Here's how the part is built. I have some questions about the finished solid (model axes, mm). Face numbers are marked on the shaded views. Round coordinates to 2 decimals unless told otherwise and drop trailing zeros. Loops run counter-clockwise (first coordinate to the right, second up) from the corner with the lowest first, then second, coordinate; pieces in that order, holes last. Notation, with made-up numbers: M 39,52 L 77,52 A32 cw 77,83 Z; hole C 43,-18.75 d1. An arc over 180 degrees is marked long. Use a Markdown table: item, result.
```python
from build123d import *

# Parameters (mm, degrees)
F1_W     = 78
F1_H     = 78
F1_R     = 2.3
F1_R_2   = 1.25
F2_DEPTH = 1.6
F3_W     = 17
F3_H     = 17
F3_R     = 2.3
F3_R_2   = 1.25
F4_DEPTH = 5.1
F5_DEPTH = 10
F6_SIZE  = 3
F7_R     = 3
F8_SIZE  = 4
F9_DEPTH = 12.5


with BuildPart() as f2:
    # F1 (on Top) → F2 (new body, symmetric)
    with BuildSketch(Plane.XY):
        Rectangle(F1_W, F1_H)
        with Locations((-36, -34.35)):
            Circle(F1_R, mode=Mode.SUBTRACT)
        with Locations((7.7, -34.35)):
            Circle(F1_R, mode=Mode.SUBTRACT)
        with Locations((36, -34.35)):
            Circle(F1_R, mode=Mode.SUBTRACT)
        with Locations((-36, 9.35)):
            Circle(F1_R, mode=Mode.SUBTRACT)
        with Locations((7.7, 9.35)):
            Circle(F1_R, mode=Mode.SUBTRACT)
        with Locations((36, 9.35)):
            Circle(F1_R, mode=Mode.SUBTRACT)
        with Locations((0, 25.5)):
            Circle(F1_R_2, mode=Mode.SUBTRACT)
        with Locations((-36, 9.35)):
            Circle(F1_R)
        with Locations((-36, 9.35)):
            Circle(F1_R_2, mode=Mode.SUBTRACT)
        with Locations((36, 9.35)):
            Circle(F1_R)
        with Locations((36, 9.35)):
            Circle(F1_R_2, mode=Mode.SUBTRACT)
        with Locations((36, -34.35)):
            Circle(F1_R)
        with Locations((36, -34.35)):
            Circle(F1_R_2, mode=Mode.SUBTRACT)
        with Locations((-36, -34.35)):
            Circle(F1_R)
        with Locations((-36, -34.35)):
            Circle(F1_R_2, mode=Mode.SUBTRACT)
        with Locations((7.7, 9.35)):
            Circle(F1_R)
        with Locations((7.7, 9.35)):
            Circle(F1_R_2, mode=Mode.SUBTRACT)
        with Locations((7.7, -34.35)):
            Circle(F1_R)
        with Locations((7.7, -34.35)):
            Circle(F1_R_2, mode=Mode.SUBTRACT)
        with Locations((-36, 9.35)):
            Circle(F1_R_2)
        with Locations((7.7, 9.35)):
            Circle(F1_R_2)
        with Locations((36, 9.35)):
            Circle(F1_R_2)
        with Locations((-36, -34.35)):
            Circle(F1_R_2)
        with Locations((7.7, -34.35)):
            Circle(F1_R_2)
        with Locations((36, -34.35)):
            Circle(F1_R_2)
    extrude(amount=F2_DEPTH, both=True)

    # F3 (on Top) → F4 (join)
    with BuildSketch(Plane.XY):
        Rectangle(F3_W, F3_H)
        with Locations((-23.5, 0)):
            Rectangle(F3_W, F3_H)
        with Locations((23.5, 0)):
            Rectangle(F3_W, F3_H)
        with Locations((23.5, 23.5)):
            Rectangle(F3_W, F3_H)
        with Locations((-23.5, -23.5)):
            Rectangle(F3_W, F3_H)
        with Locations((0, -23.5)):
            Rectangle(F3_W, F3_H)
        with Locations((23.5, -23.5)):
            Rectangle(F3_W, F3_H)
        with Locations((-23.5, 23.5)):
            Rectangle(F3_W, F3_H)
        with Locations((-11.75, 0)):
            Circle(F3_R)
        with Locations((-11.75, 0)):
            Circle(F3_R_2, mode=Mode.SUBTRACT)
        with Locations((0, 11.75)):
            Circle(F3_R)
        with Locations((0, 11.75)):
            Circle(F3_R_2, mode=Mode.SUBTRACT)
        with Locations((11.75, 0)):
            Circle(F3_R)
        with Locations((11.75, 0)):
            Circle(F3_R_2, mode=Mode.SUBTRACT)
        with Locations((0, -11.75)):
            Circle(F3_R)
        with Locations((0, -11.75)):
            Circle(F3_R_2, mode=Mode.SUBTRACT)
        with Locations((-11.75, -23.5)):
            Circle(F3_R)
        with Locations((-11.75, -23.5)):
            Circle(F3_R_2, mode=Mode.SUBTRACT)
        with Locations((-35.25, -23.5)):
            Circle(F3_R)
        with Locations((-35.25, -23.5)):
            Circle(F3_R_2, mode=Mode.SUBTRACT)
        with Locations((11.75, -23.5)):
            Circle(F3_R)
        with Locations((11.75, -23.5)):
            Circle(F3_R_2, mode=Mode.SUBTRACT)
        with Locations((35.25, -23.5)):
            Circle(F3_R)
        with Locations((35.25, -23.5)):
            Circle(F3_R_2, mode=Mode.SUBTRACT)
        with Locations((35.25, 0)):
            Circle(F3_R)
        with Locations((35.25, 0)):
            Circle(F3_R_2, mode=Mode.SUBTRACT)
        with Locations((23.5, -11.75)):
            Circle(F3_R)
        with Locations((23.5, -11.75)):
            Circle(F3_R_2, mode=Mode.SUBTRACT)
        with Locations((-23.5, -11.75)):
            Circle(F3_R)
        with Locations((-23.5, -11.75)):
            Circle(F3_R_2, mode=Mode.SUBTRACT)
        with Locations((-35.25, 0)):
            Circle(F3_R)
        with Locations((-35.25, 0)):
            Circle(F3_R_2, mode=Mode.SUBTRACT)
        with Locations((-35.25, 23.5)):
            Circle(F3_R)
        with Locations((-35.25, 23.5)):
            Circle(F3_R_2, mode=Mode.SUBTRACT)
        with Locations((-23.5, 35.25)):
            Circle(F3_R)
        with Locations((-23.5, 35.25)):
            Circle(F3_R_2, mode=Mode.SUBTRACT)
        with Locations((-23.5, 11.75)):
            Circle(F3_R)
        with Locations((-23.5, 11.75)):
            Circle(F3_R_2, mode=Mode.SUBTRACT)
        with Locations((-11.75, 23.5)):
            Circle(F3_R)
        with Locations((-11.75, 23.5)):
            Circle(F3_R_2, mode=Mode.SUBTRACT)
        with Locations((11.75, 23.5)):
            Circle(F3_R)
        with Locations((11.75, 23.5)):
            Circle(F3_R_2, mode=Mode.SUBTRACT)
        with Locations((35.25, 23.5)):
            Circle(F3_R)
        with Locations((35.25, 23.5)):
            Circle(F3_R_2, mode=Mode.SUBTRACT)
        with Locations((23.5, 11.75)):
            Circle(F3_R)
        with Locations((23.5, 11.75)):
            Circle(F3_R_2, mode=Mode.SUBTRACT)
        with Locations((23.5, 35.25)):
            Circle(F3_R)
        with Locations((23.5, 35.25)):
            Circle(F3_R_2, mode=Mode.SUBTRACT)
        with Locations((0, 35.25)):
            Circle(F3_R)
        with Locations((0, 35.25)):
            Circle(F3_R_2, mode=Mode.SUBTRACT)
        with Locations((-23.5, -35.25)):
            Circle(F3_R)
        with Locations((-23.5, -35.25)):
            Circle(F3_R_2, mode=Mode.SUBTRACT)
        with Locations((0, -35.25)):
            Circle(F3_R)
        with Locations((0, -35.25)):
            Circle(F3_R_2, mode=Mode.SUBTRACT)
        with Locations((23.5, -35.25)):
            Circle(F3_R)
        with Locations((23.5, -35.25)):
            Circle(F3_R_2, mode=Mode.SUBTRACT)
    extrude(amount=F4_DEPTH)

    # F3 (on Top) → F5 (cut, symmetric)
    with BuildSketch(Plane.XY):
        with Locations((-23.5, 23.5)):
            Rectangle(F3_W, F3_H)
        with Locations((23.5, 23.5)):
            Rectangle(F3_W, F3_H)
        with Locations((23.5, 0)):
            Rectangle(F3_W, F3_H)
        Rectangle(F3_W, F3_H)
        with Locations((-23.5, 0)):
            Rectangle(F3_W, F3_H)
        with Locations((-23.5, -23.5)):
            Rectangle(F3_W, F3_H)
        with Locations((0, -23.5)):
            Rectangle(F3_W, F3_H)
        with Locations((23.5, -23.5)):
            Rectangle(F3_W, F3_H)
    extrude(amount=F5_DEPTH, both=True, mode=Mode.SUBTRACT)

    # F6
    f6_edges = [f2.edges().sort_by_distance(p)[0] for p in [
        (39, 39, 0),
        (-39, 39, 0),
    ]]
    chamfer(f6_edges, length=F6_SIZE)

    # F7
    f7_edges = [f2.edges().sort_by_distance(p)[0] for p in [
        (-39, -39, 0),
        (39, -39, 0),
    ]]
    fillet(f7_edges, radius=F7_R)

    # F8
    f8_edges = [f2.edges().sort_by_distance(p)[0] for p in [
        (8.5, 8.5, 0),
        (-8.5, -8.5, 0),
        (8.5, -32, 0),
    ]]
    chamfer(f8_edges, length=F8_SIZE)

    # F1 (on Top) → F9 (cut, symmetric)
    with BuildSketch(Plane.XY):
        with Locations((7.7, 9.35)):
            Circle(F1_R_2)
        with Locations((-36, 9.35)):
            Circle(F1_R_2)
        with Locations((-36, -34.35)):
            Circle(F1_R_2)
        with Locations((7.7, -34.35)):
            Circle(F1_R_2)
        with Locations((36, 9.35)):
            Circle(F1_R_2)
        with Locations((36, -34.35)):
            Circle(F1_R_2)
    extrude(amount=F9_DEPTH, both=True, mode=Mode.SUBTRACT)


solid = f2.part
```
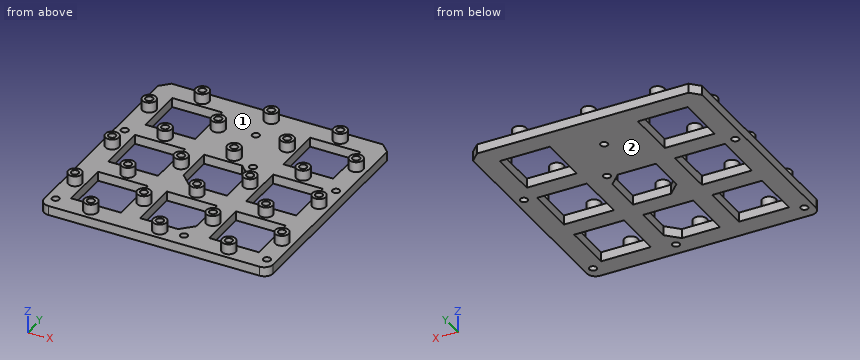
Q1. I need wall thicknesses on line 1 (Y direction, x = -24.5, z = -0.75); line 2 (Y direction, x = -11.75, z = 2.85); line 3 (Y direction, x = 3.5, z = 1). Which ranges of each line are inside material? Lowest first, please. Write a range as from..to.
Return value:
| item | result |
|---|---|
| line 1 | y = -39..-32, -15..-8.5, 8.5..15, 32..39 |
| line 2 | y = -25.8..-24.75, -22.25..-21.2, -2.3..-1.25, 1.25..2.3, 21.2..22.25, 24.75..25.8 |
| line 3 | y = -39..-32, -15..-8.5, 8.5..39 |
Q2. Imagine slicing it at C-C, the plane y = 16. Please give me the cut outline in (x, z).
Return value:
| item | result |
|---|---|
| outline | M -39,-1.6 L -32,-1.6 L -32,1.6 L -39,1.6 Z; M -15,-1.6 L 15,-1.6 L 15,1.6 L -15,1.6 Z; M 32,-1.6 L 39,-1.6 L 39,1.6 L 32,1.6 Z |
Q3. Imagine slicing it at A-A, the plane y = -16. Please give me the cut outline in (x, z), then the cut area to 3 significant figures.
Return value:
| item | result |
|---|---|
| outline | M -39,-1.6 L -32,-1.6 L -32,1.6 L -39,1.6 Z; M -15,-1.6 L -8.5,-1.6 L -8.5,1.6 L -15,1.6 Z; M 8.5,-1.6 L 15,-1.6 L 15,1.6 L 8.5,1.6 Z; M 32,-1.6 L 39,-1.6 L 39,1.6 L 32,1.6 Z |
| area | 86.4 mm^2 |
Q4. Imagine slicing it at D-D, the plane z = 4. Give the number of separate pieces and of enclosed holes in the cut face, then the cut area to 3 significant figures.
Return value:
| item | result |
|---|---|
| separate pieces | 24 |
| enclosed holes | 24 |
| area | 281 mm^2 |
Q5. Will this pin go through, and if not, where does the flat tip stop? P1, Ø3, axis at x = 36, y = -34.35, coming from the +Z side.
Return value:
| item | result |
|---|---|
| P1 | stops at z = 1.6 |
Q6. We'd pull the mould along X, two halves only. Please class the marked faces 1 and 2: pulls with the +X half, pulls with the -X half, needs draft (parallel to the pull), parting line crosses it, or undercut.
Return value:
| item | result |
|---|---|
| face 1 | undercut |
| face 2 | needs draft |
